The listing builds one solid part. Answer for the finished solid, in the listing's coordinates (mm). Face numbers are marked on the shaded views. A direction names the side the tool comes from. Give positions to 0.01 mm unless a question says otherwise; leave off trailing zeros. Order: outer loops, then holes, each group sorted by start corner. A loop starts at its lowest first (then second) coordinate and runs counter-clockwise, first axis right, second up.
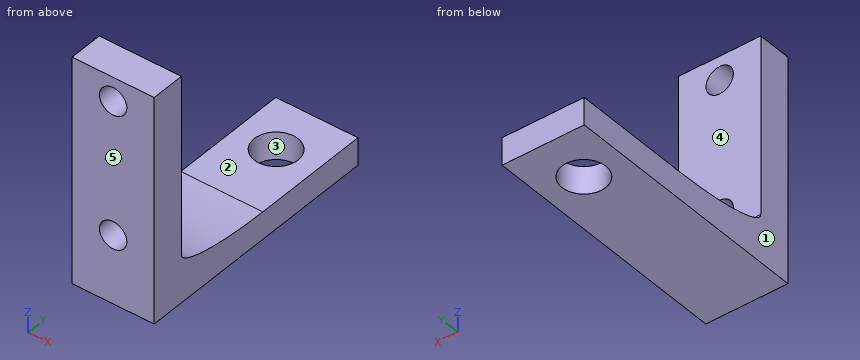
```python
from build123d import *

# Parameters (mm, degrees)
SKETCH1_W           = 12
SKETCH1_H           = 32.5
SKETCH1_R           = 3.2
BOSS_EXTRUDE1_DEPTH = 4
SKETCH2_W           = 12
SKETCH2_H           = 33
SKETCH2_R           = 2
BOSS_EXTRUDE2_DEPTH = 5
FILLET1_SIZE        = 15
FILLET1_SIZE_2      = 3


with BuildPart() as part:
    # Sketch1 → Boss-Extrude1 (new body)
    with BuildSketch(Plane.XY):
        with Locations((6, 16.25)):
            Rectangle(SKETCH1_W, SKETCH1_H)
        with Locations((6, 25)):
            Circle(SKETCH1_R, mode=Mode.SUBTRACT)
    extrude(amount=BOSS_EXTRUDE1_DEPTH)

    # Sketch2 → Boss-Extrude2 (add)
    with BuildSketch(Plane.XZ):
        with Locations((6, 16.5)):
            Rectangle(SKETCH2_W, SKETCH2_H)
        with Locations(Location((6, 10, 0), (0, 0, 270))):
            Circle(SKETCH2_R, mode=Mode.SUBTRACT)
        with Locations(Location((6, 29.5, 0), (0, 0, 270))):
            Circle(SKETCH2_R, mode=Mode.SUBTRACT)
    extrude(amount=BOSS_EXTRUDE2_DEPTH)

    # Fillet1
    # an asymmetric fillet: 15, 3 mm, written as the material it adds along each edge
    with BuildSketch(Plane(origin=(0, 0, 4), x_dir=(0, 1, 0), z_dir=(1, 0, 0))) as fillet1_piece_1:
        with BuildLine():
            Bezier((FILLET1_SIZE, 0), (0, 0), (0, FILLET1_SIZE_2), weights=[1, 0.707106781, 1])
            Line((0, FILLET1_SIZE_2), (0, 0))
            Line((0, 0), (FILLET1_SIZE, 0))
        make_face()
    extrude(amount=12)


solid = part.part
```
1) Find section C-C (z = 2.5). Write down the section's boundary in (x, y), then the cut area to 3 significant figures.
Geometry says:
outline: (0, -5) - (12, -5) - (12, 32.5) - (0, 32.5) - close; hole circle Ø6.4 at (6, 25)
area: 418 mm2
2) Straight lines are drawn through the part: probe 1 along X at (y, z) = (-3.05, 10); probe 2 along Y at (x, z) = (6, 1); probe 3 along Y at (x, z) = (0.5, 28). For each, find the intervals that lie inside material, in ascending order.
Geometry says:
probe 1: x = 0 to 4, 8 to 12
probe 2: y = -5 to 21.8, 28.2 to 32.5
probe 3: y = -5 to 0
3) A tool of negligible diameter and unlimited length cuts with its end or side. For the marked faces 4 and 5, from which of +Z, -Z, +X, -X, +Y, -Y can it reach the whole face along a straight path? Write none if from no direction.
Geometry says:
face 4: +Z, +X, -X, +Y
face 5: +Z, -Z, +X, -X, -Y
4) Find section B-B (y = 25). Write down the section's boundary in (x, z), then the cut area to 3 significant figures.
Geometry says:
outline: (0, 0) - (2.8, 0) - (2.8, 4) - (0, 4) - close; (9.2, 0) - (12, 0) - (12, 4) - (9.2, 4) - close
area: 22.4 mm2
5) Given P1, Ø4, axis at x = 1.5, y = 4.5, coming from the +Z side; P2, Ø2, axis at x = 3, y = 15, coming from the +Z side; P3, Ø5, axis at x = 6, z = 29.5, coming from the +Y side, each flat-ended and moving along its own axis, determine where each tip first touches the part or whether it passes through.
Geometry says:
P1: stops at z = 5.34
P2: stops at z = 4.01
P3: stops at y = 0
6) For a pull along X with two mould halves and no side action, classify the marked faces 1, 2 and 3 as +X half, -X half, draft (parallel to the pull), parting line (faces both ways), or undercut.
Geometry says:
face 1: -X half
face 2: draft
face 3: undercut
7) Find section D-D (x = 6). Count the separate pieces of the cut face and the enclosed holes in it, then the cut area to 3 significant figures.
Geometry says:
separate pieces: 4
enclosed holes: 0
area: 239 mm2
8) Find section A-A (z = 10). Write down the section's boundary in (x, y).
Geometry says:
outline: (0, -5) - (4, -5) - (4, 0) - (0, 0) - close; (8, -5) - (12, -5) - (12, 0) - (8, 0) - close
